from build123d import *

# Parameters (mm, degrees)
SKETCH2_W           = 106
SKETCH2_H           = 71
SKETCH2_W_2         = 17
SKETCH2_H_2         = 14
SKETCH2_W_3         = 10
SKETCH2_H_3         = 7
BOSS_EXTRUDE1_DEPTH = 1.5
SKETCH3_R           = 2
CUT_EXTRUDE1_DEPTH  = 1.5
CHAMFER2_SIZE       = 0.5
SKETCH4_W           = 5
SKETCH4_H           = 30
CUT_EXTRUDE2_DEPTH  = 1.5
FILLET1_R           = 0.5


# Read off the part's stored shape, not the designer's step: Mirror1
with BuildPart() as part:
    # Sketch2 → Boss-Extrude1 (new body)
    with BuildSketch(Plane(origin=(0, 0, 0), x_dir=(1, 0, 0), z_dir=(0, 1, 0))):
        Rectangle(SKETCH2_W, SKETCH2_H)
        with Locations((34.5, -20)):
            Rectangle(SKETCH2_W_2, SKETCH2_H_2, mode=Mode.SUBTRACT)
        with Locations((-38.5, -20)):
            Rectangle(SKETCH2_W_2, SKETCH2_H_2, mode=Mode.SUBTRACT)
        with Locations((6.5, 26.5)):
            Rectangle(SKETCH2_W_3, SKETCH2_H_3, mode=Mode.SUBTRACT)
    extrude(amount=BOSS_EXTRUDE1_DEPTH)

    # Sketch3 → Cut-Extrude1 (cut)
    with BuildSketch(Plane(origin=(0, 1.5, 0), x_dir=(1, 0, 0), z_dir=(0, 1, 0))):
        with Locations(Location((49.5, 32, 0), (0, 0, 270))):
            Circle(SKETCH3_R)
    extrude(amount=-CUT_EXTRUDE1_DEPTH, mode=Mode.SUBTRACT)

    # Chamfer2
    chamfer2_edges = [part.edges().sort_by_distance(p)[0] for p in [
        (49.5, 1.5, -34),
    ]]
    chamfer(chamfer2_edges, length=CHAMFER2_SIZE)

    # Mirror1 outline → Mirror1 (revolve, cut)
    with BuildSketch(Plane(origin=(-49.5, 0, 32), x_dir=(1, 0, 0), z_dir=(0, 0, 1))):
        Polygon((0, 0), (2, 0), (2, 1), (2.5, 1.5), (0, 1.5), align=None)
    revolve(axis=Axis((-49.5, 0, 32), (0, 1, 0)), mode=Mode.SUBTRACT)

    # Mirror1 2 outline → Mirror1 2 (revolve, cut)
    with BuildSketch(Plane(origin=(49.5, 0, 32), x_dir=(1, 0, 0), z_dir=(0, 0, 1))):
        Polygon((0, 0), (2, 0), (2, 1), (2.5, 1.5), (0, 1.5), align=None)
    revolve(axis=Axis((49.5, 0, 32), (0, 1, 0)), mode=Mode.SUBTRACT)

    # Mirror1 3 outline → Mirror1 3 (revolve, cut)
    with BuildSketch(Plane(origin=(-49.5, 0, -32), x_dir=(1, 0, 0), z_dir=(0, 0, 1))):
        Polygon((0, 0), (2, 0), (2, 1), (2.5, 1.5), (0, 1.5), align=None)
    revolve(axis=Axis((-49.5, 0, -32), (0, 1, 0)), mode=Mode.SUBTRACT)

    # Sketch4 → Cut-Extrude2 (cut)
    with BuildSketch(Plane(origin=(0, 1.5, 0), x_dir=(1, 0, 0), z_dir=(0, 1, 0))):
        with Locations((-50.5, 13)):
            Rectangle(SKETCH4_W, SKETCH4_H)
    extrude(amount=-CUT_EXTRUDE2_DEPTH, mode=Mode.SUBTRACT)

    # Fillet1
    fillet1_edges = [part.edges().sort_by_distance(p)[0] for p in [
        (53, 0.75, 35.5),
        (-53, 0.75, 35.5),
        (-53, 0.75, -35.5),
        (53, 0.75, -35.5),
        (-53, 0.75, 2),
        (-53, 0.75, -28),
        (-48, 0.75, -28),
        (-48, 0.75, 2),
    ]]
    fillet(fillet1_edges, radius=FILLET1_R)


solid = part.part
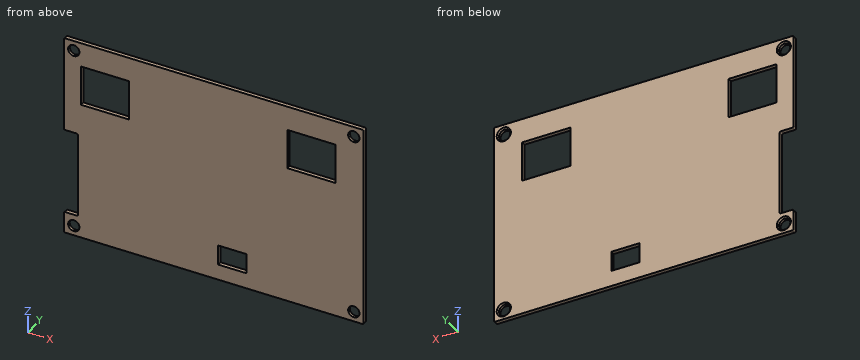
Can you work these out from the model? Positions are in its coordinate system, mm. Round coordinates to 2 decimals unless told otherwise and drop trailing zeros. Loops run counter-clockwise (first coordinate to the right, second up) from the corner with the lowest first, then second, coordinate; pieces in that order, holes last. Notation, with made-up numbers: (-5.5, -3.5) - (44.5, -3.5) arc R20 ccw to (44.5, 11.5) - close; hole circle Ø11 at (-32.5, -27). An arc over 180 degrees is marked (long way). Use CSV: the item, a comma, the result in double quotes. Start each with the question number.
1) Please list where these lines run through material, in increasing order: probe 1 along X at (y, z) = (0.4, 32); probe 2 along X at (y, z) = (1.1, 15); probe 3 along Z at (x, y) = (-49.5, 0.6). Write a range as [from, to].
2) If we section it at D-D on x = 30: Write out the boundary of the cut face in (y, z).
3) If we section it at A-A on z = 32: Write out the boundary of the cut face in (x, y).
4) If we section it at C-C on x = 49.5: Write out the boundary of the cut face in (y, z), plus the area to 3 significant figures.
5) For pin 1 Ø3 at (x, z) = (-49.5, 32) entering from +Y, with a flat end and sliding along its axis, tell me the tip position at first contact or that it passes through.
6) If we section it at B-B on y = 0.65: Count the separate pieces of the cut face and the enclosed holes in it, plus the area to 3 significant figures.
Geometry results:
1,probe 1,"x = [-53, -51.5], [-47.5, 47.5], [51.5, 53]"
1,probe 2,"x = [-53, -47], [-30, 26], [43, 53]"
1,probe 3,"z = [-35.5, -34], [-30, -28], [2, 30], [34, 35.5]"
2,outline,"(0, -35.5) - (1.5, -35.5) - (1.5, 13) - (0, 13) - close; (0, 27) - (1.5, 27) - (1.5, 35.5) - (0, 35.5) - close"
3,outline,"(-53, 0) - (-51.5, 0) - (-51.5, 1) - (-52, 1.5) - (-53, 1.5) - close; (-47.5, 0) - (47.5, 0) - (47.5, 1) - (47, 1.5) - (-47, 1.5) - (-47.5, 1) - close; (51.5, 0) - (53, 0) - (53, 1.5) - (52, 1.5) - (51.5, 1) - close"
4,outline,"(0, -35.5) - (1.5, -35.5) - (1.5, -34.5) - (1, -34) - (0, -34) - close; (0, -30) - (1, -30) - (1.5, -29.5) - (1.5, 29.5) - (1, 30) - (0, 30) - close; (0, 34) - (1, 34) - (1.5, 34.5) - (1.5, 35.5) - (0, 35.5) - close"
4,area,"94.0 mm2"
5,pin 1,"passes through"
6,separate pieces,"1"
6,enclosed holes,"7"
6,area,"6,780 mm2"
